Autodesk Inventor part; units mm, degrees
ref_plane "YZ Plane" through (0, 0, 0) normal (1, 0, 0) x (0, 1, 0)
ref_plane "XZ Plane" through (0, 0, 0) normal (0, 1, 0) x (-1, 0, 0)
ref_plane "XY Plane" through (0, 0, 0) normal (0, 0, 1) x (1, 0, 0)
sketch "スケッチ1" plane through (0, 0, 0) normal (0, 0, 1) x (1, 0, 0)
  circle A0 centre (0, 0) radius 17.9
  circle A1 centre (0, 0) radius 19.25
  line L0 (0, 0) -> (1.25, 19.2094)
  line L1 (0, 0) -> (-1.25, 19.2094)
  line L2 (0, -26.95) -> (0, 26.95)
  point P0 (1.1623, 17.8622)
  point P1 (-1.1623, 17.8622)
  dimension "d0" = 35.8
  dimension "d1" = 38.5
  dimension "d4" = 2.5
extrude "押し出し1" add sketch "スケッチ1" along normal blind 38 contours A0 L0 A1 L2 | L2 A1 L1 A0 picked at (1.4278, -18.6391) picked at (-2.7104, 18.4842)
sketch "スケッチ2" plane through (0, 0, 38) normal (0, 0, 1) x (1, 0, 0)
  line L0 (0, 0) -> (-19.224, -1)
  arc A0 (-1.25, 19.2094) -> (1.25, 19.2094) centre (0, 0) ccw
  line L1 (0, 0) -> (-19.224, 1)
  line L2 (-26.95, 0) -> (26.95, 0)
  arc A1 (-18.3752, 0.9558) -> (-18.3752, -0.9558) centre (0, 0) ccw
  arc A2 (-1.1623, 17.8622) -> (1.1623, 17.8622) centre (0, 0) ccw
  dimension "d5" = 2
  dimension "d6" = 0.5
extrude "押し出し2" cut sketch "スケッチ2" against normal blind 2 contours L0 A0 L2 A1 | L2 A0 L1 A1
fillet "フィレット1" radius 0.5 3 edges at (-19.25, 0, 36) (-19.224, -1, 37) (-19.224, 1, 37)
sketch "スケッチ3" plane through (0, 0, 0) normal (0, 1, 0) x (-1, 0, 0)
  line L0 (-18, 30) -> (18, 30)
  line L1 (18, 30) -> (18, 10.5)
  line L2 (18, 10.5) -> (-18, 10.5)
  line L3 (-18, 10.5) -> (-18, 30)
  line L4 (19.1905, 38) -> (-19.25, 38)
  point P0 (0, 0)
  point P1 (-1.25, 38)
  point P2 (0, 10.5)
  dimension "d10" = 8
  dimension "d11" = 19.5
  dimension "d12" = 36
sketch3d "3D スケッチ1"
split_face "分割1"
fillet "フィレット2" radius 0.1 2 edges at (-1.25, 19.2094, 19) (1.25, 19.2094, 19)
properties part number "555_Outer" material "鉄、鋳鉄"
Build history of the part. All positions in model axes, mm. A direction names the side the tool comes from. Coordinates: 2 decimals unless noted, no trailing zeros. Write each loop counter-clockwise with the first axis right and the second up, starting at its lowest first coordinate (ties: lowest second). Pieces come first, ordered by that corner, then holes.
1. 3-axis set-ups, long thin cutter, end or side, ignore diameter. For faces 1 (the flat face through (-1.202, 18.477, 18.734)), 2 (the flat face through (-16, 9, 38)): which of +Z, -Z, +X, -X, +Y, -Y reach the whole face in a straight line?
Answer block:
face 1: +Z, -Z, +Y
face 2: +Z, +X, -X, +Y, -Y
2. Band-saw the part on A-A, the plane y = 5.5. Give the cut face in (x, z).
Answer block:
outline: (-18.45, 0) - (-17.03, 0) - (-17.03, 38) - (-18.45, 38) - close; (17.03, 0) - (18.45, 0) - (18.45, 38) - (17.03, 38) - close
3. Band-saw the part on D-D, the plane x = 0. Give the cut face in (y, z).
Answer block:
outline: (-19.25, 0) - (-17.9, 0) - (-17.9, 38) - (-19.25, 38) - close
4. Drop flat-ended pins along their axis: pin 1 (8 mm diameter, centred on x = -12, z = 31, fed in from +Y); pin 2 (4 mm diameter, centred on x = -10.5, y = -10, fed in from -Z); pin 3 (8 mm diameter, centred on y = -6, z = 14.5, fed in from -X); pin 4 (3 mm diameter, centred on y = -8.5, z = 31.5, fed in from -X). Give the stop position or say it passes through.
Answer block:
pin 1: stops at y = 17.51
pin 2: passes through
pin 3: stops at x = -19.15
pin 4: stops at x = -17.93
5. Band-saw the part on B-B, the plane x = -5. Give the cut face in (y, z).
Answer block:
outline: (-18.59, 0) - (-17.19, 0) - (-17.19, 38) - (-18.59, 38) - close; (17.19, 0) - (18.59, 0) - (18.59, 38) - (17.19, 38) - close
6. Band-saw the part on C-C, the plane z = 3. Give the cut face in (x, y), and give its area (3 significant figures).
Answer block:
outline: (-1.35, 19.2) arc R19.25 ccw (long way) to (1.35, 19.2) arc R0.1 ccw to (1.24, 19.11) - (1.16, 17.86) arc R17.9 cw (long way) to (-1.16, 17.86) - (-1.24, 19.11) arc R0.1 ccw to start
area: 154 mm2
7. Drill centre lines: probe 1 along X at (y, z) = (0, 16.5); probe 2 along X at (y, z) = (15, 32.5); probe 3 along Y at (x, z) = (-7, 30.5). Where is each one in solid material? Low to high.
Answer block:
probe 1: x = -19.25 to -17.9, 17.9 to 19.25
probe 2: x = -12.06 to -9.77, 9.77 to 12.06
probe 3: y = -17.93 to -16.47, 16.47 to 17.93
8. Pull direction Y, two halves, no side cores. Call faces 3 (the flat face through (1.202, 18.477, 18.734)), 4 (the cylindrical face through (-18.4, 0, 37)), 5 (the cylindrical face through (0.827, -19.232, 18.734)): released by +Y, released by -Y, zero draft, split by the parting line, or undercut.
Answer block:
face 3: released by +Y
face 4: undercut
face 5: split by the parting line
